Geometry: see drawing. Coordinates: mm, zero at the bounding-box minimum. Round coordinates to 2 decimals unless told otherwise and drop trailing zeros. Loops run counter-clockwise (first coordinate to the right, second up) from the corner with the lowest first, then second, coordinate; pieces in that order, holes last. Notation, with made-up numbers: (81.25, 31.5) - (134.25, 31.5) arc R17 ccw to (134.25, 45.5) - close; hole circle Ø1 at (67, 79.25). An arc over 180 degrees is marked (long way). Write item = value, one per line. Start each with the question number.
Item 1: Section A-A (z = 26.5). Return loops of the section in (x, y), plus the area to 3 significant figures.
Item 2: Section B-B (x = 50.5). Return loops of the section in (y, z).
Item 3: First-contact query: pin 1 (4 mm diameter, centred on x = 7.5, z = 51.5, fed in from +Y). Flat tip, straight axial feed; report the tip coordinate or a pass-through.
Item 4: Line query: line 1 (Z direction, x = 67.5, y = 2.1); line 2 (X direction, y = 0.75, z = 51.5); line 3 (X direction, y = 0.75, z = 34.5). Output: solid intervals per line, ascending. Write a range as from..to.
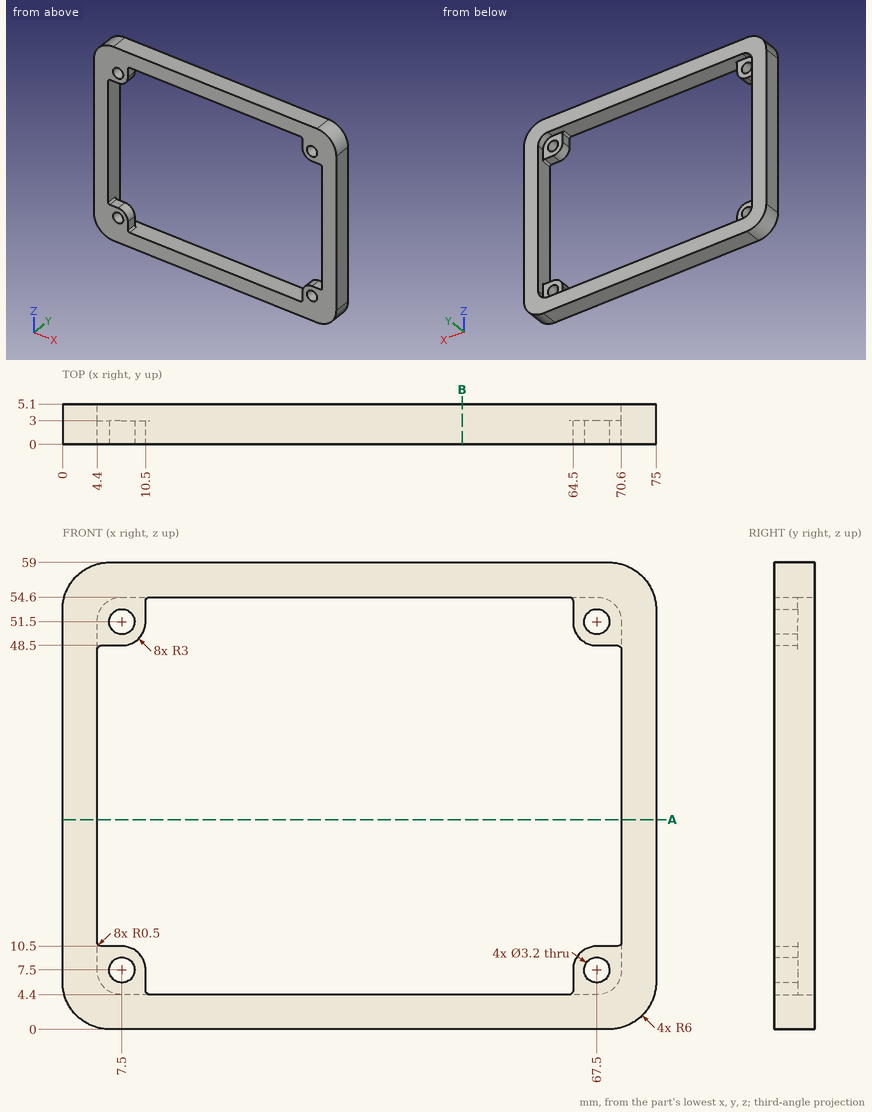
Taken from the geometry:
q1.outline = (0, 0) - (4.4, 0) - (4.4, 5.1) - (0, 5.1) - close; (70.6, 0) - (75, 0) - (75, 5.1) - (70.6, 5.1) - close
q1.area = 44.9 mm^2
q2.outline = (0, 0) - (5.1, 0) - (5.1, 4.4) - (0, 4.4) - close; (0, 54.6) - (5.1, 54.6) - (5.1, 59) - (0, 59) - close
q3.pin_1 = 3
q4.line_1 = 0..5.9, 9.1..10.5, 48.5..49.9, 53.1..59
q4.line_2 = 0..5.9, 9.1..10.5, 64.5..65.9, 69.1..75
q4.line_3 = 0..4.4, 70.6..75
